Model file for the job. Use its own axes, mm. A direction names the side the tool comes from. Coordinates: 2 decimals unless noted, no trailing zeros. Order: outer loops, then holes, each group sorted by start corner. A loop starts at its lowest first (then second) coordinate and runs counter-clockwise, first axis right, second up.
from build123d import *

# Parameters (mm, degrees)
F0_R     = 19.05
F1_DEPTH = 66.675
F3_DEPTH = 6.35
F4_R     = 2.38125
F5_DEPTH = 25.4


with BuildPart() as f1:
    # F0 (on Top) → F1 (new body)
    with BuildSketch(Plane.XY):
        Circle(F0_R)
    extrude(amount=F1_DEPTH)

    # F2 (on face) → F3 (join)
    with BuildSketch(Plane.XY.offset(66.675)):
        with BuildLine():
            ThreePointArc((7.636474, -6.945197), (5.225781, -1.964799), (-0.175923, -0.765885))
            Line((-0.175923, -0.765885), (2.748871, -13.124509))
            ThreePointArc((2.748871, -13.124509), (6.266871, -10.884504), (7.636474, -6.945197))
        make_face()
        with BuildLine():
            Line((2.748871, -13.124509), (-0.175923, -0.765885))
            ThreePointArc((-0.175923, -0.765885), (-4.892838, -8.407594), (2.748871, -13.124509))
        make_face()
    extrude(amount=F3_DEPTH)

    # F4 (on face) → F5 (join)
    with BuildSketch(Plane.XY.offset(73.025)):
        with Locations((1.286474, -6.945197)):
            Circle(F4_R)
    extrude(amount=F5_DEPTH)


solid = f1.part
Q1. Cut at D-D, the plane y = -5.5. List the corners of the cut face in (x, z) (3 decimals), plus the area to 3 significant figures.
Established:
outline: (-18.239, 0) - (18.239, 0) - (18.239, 66.675) - (7.47, 66.675) - (7.47, 73.025) - (3.179, 73.025) - (3.179, 98.425) - (-0.606, 98.425) - (-0.606, 73.025) - (-4.897, 73.025) - (-4.897, 66.675) - (-18.239, 66.675) - close
area: 2,610 mm2
Q2. Cut at B-B, the plane z = 32.5. List the corners of the cut face in (x, y), plus the area to 3 significant figures.
Established:
outline: circle Ø38.1 at (0, 0)
area: 1,140 mm2
Q3. Cut at C-C, the plane x = 9.5. List the corners of the cut face in (y, z) (3 decimals).
Established:
outline: (-16.512, 0) - (16.512, 0) - (16.512, 66.675) - (-16.512, 66.675) - close
Q4. Probe line 1 (Z direction, x = 2.5, y = 10) (3 decimals); line 2 (Y direction, x = 0.5, z = 32); line 3 (Y direction, x = 5, z = 71.5). List the from-to ranges inside material, lowest first.
Established:
line 1: z = 0 to 66.675
line 2: y = -19.04 to 19.04
line 3: y = -12.1 to -1.79
Q5. Which spindle directions (+Z, -Z, +X, -X, +Y, -Y) get a long thin tool onto all of the face, cutting with end or side? Do faces 1 (the face through (0, 0, 0)), 2 (the face through (4, -7, 73.025)). Say none if no direction does.
Established:
face 1: -Z, +X, -X, +Y, -Y
face 2: +Z
Q6. Drop flat-ended pins along their axis: P1, Ø8, axis at x = 11, y = 10, coming from the +Z side (3 decimals); P2, Ø4, axis at y = -12, z = 35, coming from the -X side; P3, Ø5, axis at x = 8, z = 44, coming from the +Y side. Give the stop position or say it passes through.
Established:
P1: stops at z = 66.675
P2: stops at x = -16.21
P3: stops at y = 18.24
Q7. Cut at A-A, the plane y = -11. List the corners of the cut face in (x, z) (3 decimals).
Established:
outline: (-15.553, 0) - (15.553, 0) - (15.553, 66.675) - (6.173, 66.675) - (6.173, 73.025) - (-3.6, 73.025) - (-3.6, 66.675) - (-15.553, 66.675) - close
